Geometry check sheet. Reference: the model listing, model coordinates, mm. Face numbers are marked on the shaded views. A direction names the side the tool comes from. Round coordinates to 2 decimals unless told otherwise and drop trailing zeros. Loops run counter-clockwise (first coordinate to the right, second up) from the corner with the lowest first, then second, coordinate; pieces in that order, holes last. Notation, with made-up numbers: M -22.75,-28 L 24.25,-28 A11 cw 24.25,-19 Z; hole C -36.5,-21.75 d4. An arc over 180 degrees is marked long. Use one line per item in the form item = value. Start each with the question number.
1. Cross-section at A-A (x = 6.5). Record the boundary of the cut face in (y, z), then the cut area to 3 significant figures.
2. Material ranges on line 1 (Y direction, x = 7, z = 14.5); line 2 (Y direction, x = -8, z = 8); line 3 (Y direction, x = -33.5, z = 16), recorded low to high.
3. Set-up check for the marked faces 1 and 2: record each of +Z, -Z, +X, -X, +Y, -Y from which the full face is reachable in a straight line by a thin tool's end or side.
4. Cross-section at D-D (x = -38). Record the boundary of the cut face in (y, z).
5. Cross-section at C-C (y = -3.5). Record the boundary of the cut face in (x, z).
6. Cross-section at B-B (z = 13). Record the boundary of the cut face in (x, y).
7. Go/stop test with flat-tipped pins: pin 1 (7 mm diameter, centred on x = 5, z = 15, fed in from -Y); pin 2 (2 mm diameter, centred on y = -32, z = 21.5, fed in from +X); pin 3 (5 mm diameter, centred on x = -30.5, y = -0.5, fed in from -Z); pin 4 (3 mm diameter, centred on y = -3, z = 18, fed in from -X). Record where each tip stops, or that it passes through.
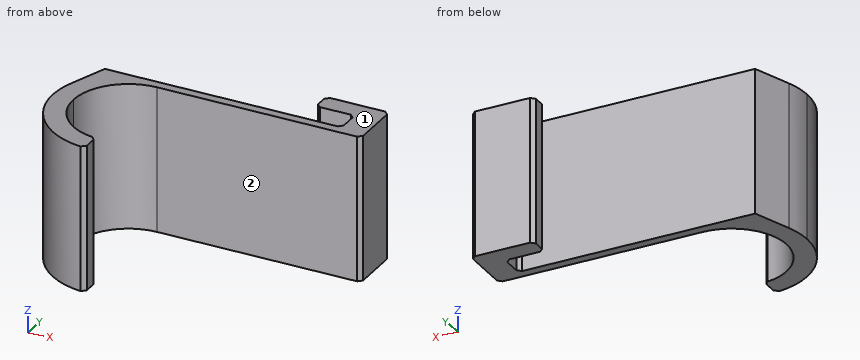
```python
from build123d import *

# Parameters (mm, degrees)
F1_DEPTH    = 30
F2_T1_DEPTH = 30
F2_T3_DEPTH = 34.1146927807
F2_T5_DEPTH = 34.5796675935
F2_T7_DEPTH = 33.7107882322


# Not quite as in the source:
# - a fillet or chamfer that OpenCascade refuses, or shapes differently, is made with other operations: its cross-section is extruded or revolved along the edge and cut away or added


with BuildPart() as f1:
    # F0 (on Top) → F1 (new body)
    with BuildSketch(Plane.XY):
        with BuildLine():
            Line((0, 4), (0, 0))
            Line((0, 0), (8, 0))
            Line((8, 0), (8, -5.11398))
            Line((8, -5.11398), (0, -5.11398))
            Line((0, -5.11398), (-30, -5.11398))
            Line((-30, -5.11398), (-40.9191332404, -5.11398))
            Line((-40.9191332404, -5.11398), (-43.7934957599, -13.012435493))
            ThreePointArc((-43.7934957599, -13.012435493), (-44.486999636, -15.5813060668), (-44.7341086379, -18.230641982))
            ThreePointArc((-44.7341086379, -18.230641982), (-40.5087550106, -29.0303309912), (-30, -33.9347131233))
            Line((-30, -33.9347131233), (-30, -29.6540509196))
            ThreePointArc((-30, -29.6540509196), (-37.4863926883, -26.0077839606), (-40.4625312712, -18.230641982))
            ThreePointArc((-40.4625312712, -18.230641982), (-37.1000637613, -10.2912492126), (-29.125629618, -7.0127517826))
            Line((-29.125629618, -7.0127517826), (0, -7.0127517826))
            Line((0, -7.0127517826), (13, -7.0127517826))
            Line((13, -7.0127517826), (13, 4))
            Line((13, 4), (0, 4))
        make_face()
    extrude(amount=F1_DEPTH)

    # F2: chamfer of 0.8 on 8 edges, made by hand

    # F2_s2 → F2_t1 (join)
    with BuildSketch(Plane.XY):
        Polygon((8, -0.8), (7.2, 0), (8, 0), align=None)
        Polygon((7.2, -5.11398), (8, -4.31398), (8, -5.11398), align=None)
    extrude(amount=F2_T1_DEPTH)

    # F2_s4 → F2_t3 (cut)
    with BuildSketch(Plane.XY.offset(-2.0573463904)):
        Polygon((0, 0.8), (0.8, 0), (0, 0), align=None)
        Polygon((0.8, 4), (0, 3.2), (0, 4), align=None)
        Polygon((12.2, -7.0127517826), (13, -6.2127517826), (13, -7.0127517826), align=None)
        Polygon((13, 3.2), (12.2, 4), (13, 4), align=None)
    extrude(amount=F2_T3_DEPTH, mode=Mode.SUBTRACT)

    # F2_s6 → F2_t5 (cut)
    with BuildSketch(Plane.XY.offset(-2.2898337967)):
        with BuildLine():
            Line((-30.8904518842, -33.859131698), (-30, -33.0642616101))
            Line((-30, -33.0642616101), (-30, -33.9347131233))
            ThreePointArc((-30, -33.9347131233), (-30.4567158355, -33.9023630924), (-30.8904518842, -33.859131698))
        make_face()
    extrude(amount=F2_T5_DEPTH, mode=Mode.SUBTRACT)

    # F2_s8 → F2_t7 (cut)
    with BuildSketch(Plane.XY.offset(-1.8553941161)):
        with BuildLine():
            Line((-30, -30.3717734146), (-30.6896401509, -29.5794220382))
            ThreePointArc((-30.6896401509, -29.5794220382), (-30.3570806998, -29.6207408817), (-30, -29.6540509196))
            Line((-30, -29.6540509196), (-30, -30.3717734146))
        make_face()
    extrude(amount=F2_T7_DEPTH, mode=Mode.SUBTRACT)


solid = f1.part
```
Reported:
q1.outline = M -7.01,0 L -5.11,0 L -5.11,30 L -7.01,30 Z; M 0,0 L 4,0 L 4,30 L 0,30 Z
q1.area = 177 mm²
q2.line_1 = -7.01 to -5.11, 0 to 4
q2.line_2 = -7.01 to -5.11
q2.line_3 = -33.33 to -28.81, -7.89 to -5.11
q3.face_1 = +Z, +X, -X, +Y, -Y
q3.face_2 = +Z, -Z, +X, -Y
q4.outline = M -31.19,0 L -25.41,0 L -25.41,30 L -31.19,30 Z; M -11.29,0 L -5.11,0 L -5.11,30 L -11.29,30 Z
q5.outline = M 8,0 L 13,0 L 13,30 L 8,30 Z
q6.outline = M -43.79,-13.01 A15.61 ccw -30.89,-33.86 L -30,-33.06 L -30,-30.37 L -30.69,-29.58 A11.34 cw -29.13,-7.01 L 12.2,-7.01 L 13,-6.21 L 13,3.2 L 12.2,4 L 0.8,4 L 0,3.2 L 0,0.8 L 0.8,0 L 7.2,0 L 8,-0.8 L 8,-4.31 L 7.2,-5.11 L -40.92,-5.11 Z
q7.pin_1 = -7.01
q7.pin_2 = -30
q7.pin_3 = through
q7.pin_4 = 7.81
